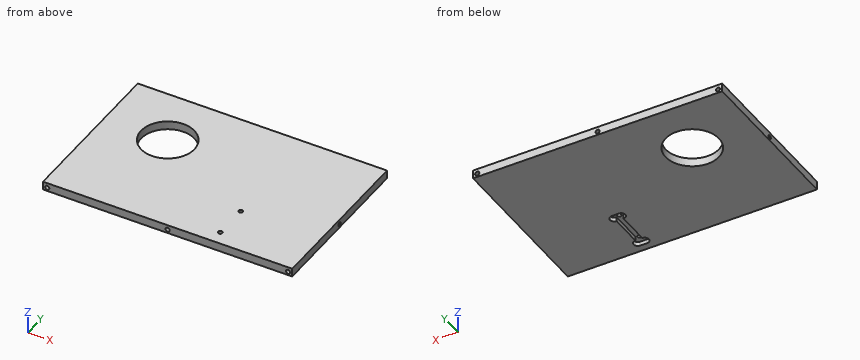
```python
from build123d import *

# Parameters (mm, degrees)
F0_R      = 19
F1_DEPTH  = 6
F2_START  = 3
F0_R_2    = 1.5
F2_DEPTH  = 3
F3_R      = 1.5
F4_DEPTH  = 8
F5_R      = 1.5
F6_DEPTH  = 8
F7_R      = 1.5
F8_DEPTH  = 5
F9_R      = 1.5
F10_DEPTH = 5


# Not quite as in the source:
# - a feature names something its author has since deleted; it is built from what else it names


with BuildPart() as f1:
    # F0 (on Top) → F1 (new body)
    with BuildSketch(Plane.XY):
        Polygon((0, 116.25), (0, 0), (177.5, 0), (177.5, 5), (177.5, 40), (177.5, 52.125), (177.5, 64.125), (177.5, 116.25), align=None)
        with BuildLine():
            ThreePointArc((123, 40), (126, 37), (123, 34))
            Line((123, 34), (123, 11))
            ThreePointArc((123, 11), (126, 8), (123, 5))
            Line((123, 5), (118, 5))
            ThreePointArc((118, 5), (115, 8), (118, 11))
            Line((118, 11), (118, 34))
            ThreePointArc((118, 34), (115, 37), (118, 40))
            Line((118, 40), (123, 40))
        make_face(mode=Mode.SUBTRACT)
        with Locations((45, 75.5)):
            Circle(F0_R, mode=Mode.SUBTRACT)
    extrude(amount=F1_DEPTH)

    # F0 (on Top) → F2 (join)
    with BuildSketch(Plane.XY.offset(F2_START)):
        with BuildLine():
            Line((123, 11), (123, 34))
            ThreePointArc((123, 34), (126, 37), (123, 40))
            Line((123, 40), (118, 40))
            ThreePointArc((118, 40), (115, 37), (118, 34))
            Line((118, 34), (118, 11))
            ThreePointArc((118, 11), (115, 8), (118, 5))
            Line((118, 5), (123, 5))
            ThreePointArc((123, 5), (126, 8), (123, 11))
        make_face()
        with Locations((120.5, 10)):
            Circle(F0_R_2, mode=Mode.SUBTRACT)
        with Locations((120.5, 35)):
            Circle(F0_R_2, mode=Mode.SUBTRACT)
    extrude(amount=F2_DEPTH)

    # F3 (on face) → F4 (cut)
    with BuildSketch(Plane.YZ.offset(177.5)):
        with Locations((58.125, 2.5)):
            Circle(F3_R)
    extrude(amount=-F4_DEPTH, mode=Mode.SUBTRACT)

    # F5 (on face) → F6 (cut)
    with BuildSketch(Plane(origin=(0, 0, 0), x_dir=(0, -1, 0), z_dir=(-1, 0, 0))):
        with Locations((-58.125, 2.5)):
            Circle(F5_R)
    extrude(amount=-F6_DEPTH, mode=Mode.SUBTRACT)

    # F7 (on face) → F8 (cut)
    with BuildSketch(Plane.XZ):
        with Locations((3, 2.5)):
            Circle(F7_R)
        with Locations((88.75, 2.5)):
            Circle(F7_R)
        with Locations((174.5, 2.5)):
            Circle(F7_R)
    extrude(amount=-F8_DEPTH, mode=Mode.SUBTRACT)

    # F9 (on face) → F10 (cut)
    with BuildSketch(Plane(origin=(0, 116.25, 0), x_dir=(-1, 0, 0), z_dir=(0, 1, 0))):
        with Locations((-3, 2.5)):
            Circle(F9_R)
        with Locations((-88.75, 2.5)):
            Circle(F9_R)
        with Locations((-174.5, 2.5)):
            Circle(F9_R)
    extrude(amount=-F10_DEPTH, mode=Mode.SUBTRACT)


solid = f1.part
```
The model under review builds one solid part; all positions refer to its coordinate system, in mm. Round coordinates to 2 decimals unless told otherwise and drop trailing zeros. Order: outer loops, then holes, each group sorted by start corner. A loop starts at its lowest first (then second) coordinate and runs counter-clockwise, first axis right, second up. Notation, with made-up numbers: (44.25, 88) -> (58.25, 88) arc R9 cw to (58.25, 96) -> close; hole circle Ø3 at (-19, 34). An arc over 180 degrees is marked (long way). One line per item, written item: value. Start each with the question number.
Q1. Wall thickness on line 1 (X direction, y = 112.5, z = 2.3); line 2 (Y direction, x = 120.5, z = 4.65); line 3 (Z direction, x = 88.75, y = 112.8): over which ranges is each line inside the solid? List them lowest first.
Q2. Take a section at A-A (x = 45). Write out the cut boundary in (y, z), and give its area (4 significant figures).
Q3. Clearance check with flat-ended pins moving along their axes: pin 1 Ø2.5 at (x, y) = (120.5, 10) entering from +Z; pin 2 Ø1 at (x, z) = (42, 3.5) entering from -Y; pin 3 Ø2.5 at (y, z) = (58.125, 2.5) entering from +X; pin 4 Ø0.9 at (x, z) = (88, 2.5) entering from +Y. State where each tip first meets the part, or that it passes through.
Q4. Take a section at B-B (y = 68). Write out the cut boundary in (x, z), and give its area (3 significant figures).
Reported:
1. line 1: x = 0 to 1.51, 4.49 to 87.26, 90.24 to 173.01, 175.99 to 177.5
1. line 2: y = 0 to 8.5, 11.5 to 33.5, 36.5 to 116.25
1. line 3: z = 0 to 1, 4 to 6
2. outline: (0, 0) -> (56.5, 0) -> (56.5, 6) -> (0, 6) -> close; (94.5, 0) -> (116.25, 0) -> (116.25, 6) -> (94.5, 6) -> close
2. area: 469.5 mm2
3. pin 1: passes through
3. pin 2: stops at y = 0
3. pin 3: stops at x = 169.5
3. pin 4: stops at y = 111.25
4. outline: (0, 0) -> (27.54, 0) -> (27.54, 6) -> (0, 6) -> close; (62.46, 0) -> (177.5, 0) -> (177.5, 6) -> (62.46, 6) -> close
4. area: 856 mm2
